```python
from build123d import *

# Parameters (mm, degrees)
ESQUISSE2_W             = 5.291502622
ESQUISSE2_H             = 1
ENL_V_MAT_EXTRU_1_DEPTH = 10
ESQUISSE3_R             = 1.5
FIXHOLES_DEPTH          = 3
REPEATFIXHOLES_COUNT    = 4


with BuildPart() as part:
    # Esquisse1 → MainRevolution (revolve)
    with BuildSketch(Plane.XY):
        Polygon((0, 0), (98.5, 0), (98.5, 4), (81.9, 4), (81.9, 9), (77.9, 9), (77.9, 15), (50.8, 15), (50.8, 13), (14.8, 13), (14.8, 12), (8.8, 12), (8.8, 2), (0, 2), align=None)
    revolve(axis=Axis((0, 0, 0), (1, 0, 0)))

    # Esquisse2 → Enl_v. mat.-Extru.1 (cut)
    with BuildSketch(Plane(origin=(98.5, 0, 0), x_dir=(0, 0, -1), z_dir=(1, 0, 0))):
        with Locations((0, 3.5)):
            Rectangle(ESQUISSE2_W, ESQUISSE2_H)
    extrude(amount=-ENL_V_MAT_EXTRU_1_DEPTH, mode=Mode.SUBTRACT)

    # Esquisse3 → FixHoles (cut)
    with BuildSketch(Plane(origin=(77.9, 0, 0), x_dir=(0, 0, -1), z_dir=(1, 0, 0))):
        with Locations((0, 13)):
            Circle(ESQUISSE3_R)
    fixholes = extrude(amount=-FIXHOLES_DEPTH, mode=Mode.SUBTRACT)

    # RepeatFixHoles: FixHoles ×4 about axis
    repeatfixholes_axis = Axis((0, 0, 0), (1, 0, 0))
    for i in range(1, REPEATFIXHOLES_COUNT):
        add(fixholes.rotate(repeatfixholes_axis, i * 360 / REPEATFIXHOLES_COUNT), mode=Mode.SUBTRACT)


solid = part.part
```
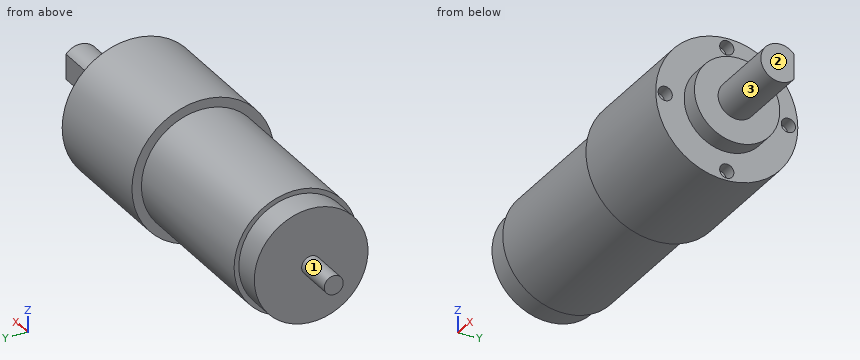
Geometry: final body of the model. Coordinates: model frame, mm. Face numbers are marked on the shaded views. A direction names the side the tool comes from. Give positions to 0.01 mm unless a question says otherwise; leave off trailing zeros. Write each loop counter-clockwise with the first axis right and the second up, starting at its lowest first coordinate (ties: lowest second). Pieces come first, ordered by that corner, then holes.
1. Line query: probe 1 along Z at (x, y) = (75.8, 0); probe 2 along X at (y, z) = (9, 7.5); probe 3 along Y at (x, z) = (64, -9). Output: solid intervals per line, ascending.
2. Section query D-D, the plane z = -7.5. Return loops of the section in (x, y), then the cut area to 3 significant figures.
3. Section query C-C, the plane x = 59.5. Return loops of the section in (y, z).
4. Pin query (flat end, axial travel): P1, Ø4, axis at x = 48.5, y = -7, coming from the -Z side; P2, Ø5, axis at y = 13, z = 0, coming from the +X side; P3, Ø3, axis at x = 16, z = -5.5, coming from the +Y side; P4, Ø9, axis at y = -3.5, z = 4, coming from the +X side. Return the tip coordinate at first contact, or that it passes through.
5. Reachability of the marked faces 1, 2 and 3 from +Z, -Z, +X, -X, +Y, -Y: full face, straight path, thin tool, end or side. Return the list, or none.
Computed:
1. probe 1: z = -15 to -14.5, -11.5 to 11.5, 14.5 to 15
1. probe 2: x = 8.8 to 77.9
1. probe 3: y = -12 to 12
2. outline: (8.8, -9.37) - (14.8, -9.37) - (14.8, -10.62) - (50.8, -10.62) - (50.8, -12.99) - (77.9, -12.99) - (77.9, -4.97) - (81.9, -4.97) - (81.9, 4.97) - (77.9, 4.97) - (77.9, 12.99) - (50.8, 12.99) - (50.8, 10.62) - (14.8, 10.62) - (14.8, 9.37) - (8.8, 9.37) - close
2. area: 1,620 mm2
3. outline: circle Ø30 at (0, 0)
4. P1: stops at z = -12
4. P2: stops at x = 77.9
4. P3: stops at y = 12.37
4. P4: stops at x = 98.5
5. face 1: -X
5. face 2: +Z, -Z, +X, +Y, -Y
5. face 3: +X
